from build123d import *

# Parameters (mm, degrees)
CYLINDER002_R     = 1.5
CYLINDER002_DEPTH = 1
CYLINDER_R        = 2
CYLINDER_DEPTH    = 4
CYLINDER001_R     = 1.5
CYLINDER001_DEPTH = 4


with BuildPart() as cylinder002:
    # Cylinder002 → Cylinder002 (new body)
    with BuildSketch(Plane.XY):
        Circle(CYLINDER002_R)
    extrude(amount=CYLINDER002_DEPTH)


with BuildPart() as cut:
    # Cylinder → Cylinder (new body)
    with BuildSketch(Plane.XY):
        Circle(CYLINDER_R)
    extrude(amount=CYLINDER_DEPTH)

    # Cut: cut Cylinder002
    add(cylinder002.part, mode=Mode.SUBTRACT)


with BuildPart() as fusion:
    # Cylinder001 → Cylinder001 (new body)
    with BuildSketch(Plane.XY.offset(4)):
        Circle(CYLINDER001_R)
    extrude(amount=CYLINDER001_DEPTH)

    # Fusion: union Cut
    add(cut.part)


solid = fusion.part
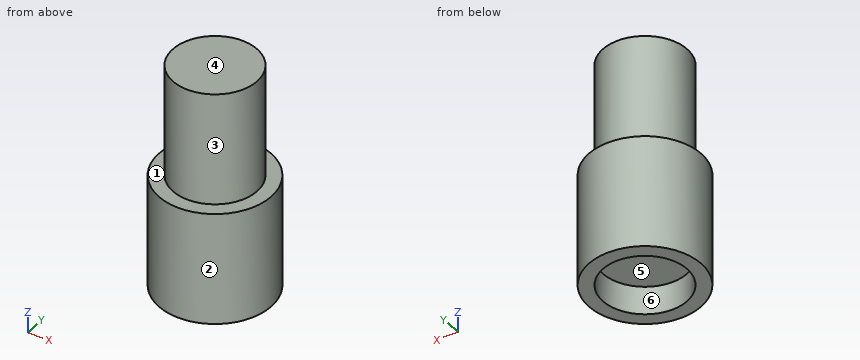
Check sheet for the modelled part. Datum: model origin and axes. Units: mm. Face numbers are marked on the shaded views. A direction names the side the tool comes from. Give positions to 0.01 mm unless a question says otherwise; leave off trailing zeros. Write each loop counter-clockwise with the first axis right and the second up, starting at its lowest first coordinate (ties: lowest second). Pieces come first, ordered by that corner, then holes. Notation, with made-up numbers: (-1, 20.5) -> (25, 20.5) arc R38 ccw to (25, 59.5) -> close; hole circle Ø1 at (14.25, 16.25). An arc over 180 degrees is marked (long way). One line per item, written item: value. Start each with the question number.
Item 1: Draft check along X on the marked faces 3, 4, 5 and 6. Enter one of: +X half, -X half, draft (parallel to the pull), parting line (faces both ways), or undercut.
Item 2: Gauge pin test, flat ends, axial feed: pin 1 (0.9 mm diameter, centred on x = 0.5, y = 0.5, fed in from -Z); pin 2 (1.5 mm diameter, centred on x = -1, z = 7, fed in from -Y). Record the tip position at first contact, or that the pin passes through.
Item 3: Section check C-C on z = 1.5. Record the cut outline in (x, y).
Item 4: Section check A-A on y = 1.2. Record the cut outline in (x, z), then the cut area to 3 significant figures.
Item 5: Section check B-B on x = 1.4. Record the cut outline in (y, z), then the cut area to 3 significant figures.
Item 6: Section check D-D on z = 7.5. Record the cut outline in (x, y), then the cut area to 3 significant figures.
Item 7: Material ranges on probe 1 along Y at (x, z) = (0, 0.85); probe 2 along Z at (x, y) = (-0.5, 0.25); probe 3 along Z at (x, y) = (0.3, -1.5), recorded low to high. Write a range as from..to.
Item 8: Tool access check on the marked faces 1 and 2. Record the directions out of +Z, -Z, +X, -X, +Y, -Y that give a thin tool (end or side, any length) a straight path to the whole face; none if there is none.
Results list:
1. face 3: parting line
1. face 4: draft
1. face 5: undercut
1. face 6: undercut
2. pin 1: z = 1
2. pin 2: y = -1.48
3. outline: circle Ø4 at (0, 0)
4. outline: (-1.6, 0) -> (-0.9, 0) -> (-0.9, 1) -> (0.9, 1) -> (0.9, 0) -> (1.6, 0) -> (1.6, 4) -> (0.9, 4) -> (0.9, 8) -> (-0.9, 8) -> (-0.9, 4) -> (-1.6, 4) -> close
4. area: 18.2 mm²
5. outline: (-1.43, 0) -> (-0.54, 0) -> (-0.54, 1) -> (0.54, 1) -> (0.54, 0) -> (1.43, 0) -> (1.43, 4) -> (0.54, 4) -> (0.54, 8) -> (-0.54, 8) -> (-0.54, 4) -> (-1.43, 4) -> close
5. area: 14.7 mm²
6. outline: circle Ø3 at (0, 0)
6. area: 7.07 mm²
7. probe 1: -2..-1.5, 1.5..2
7. probe 2: 1..8
7. probe 3: 0..4
8. face 1: +Z
8. face 2: +Z, -Z
